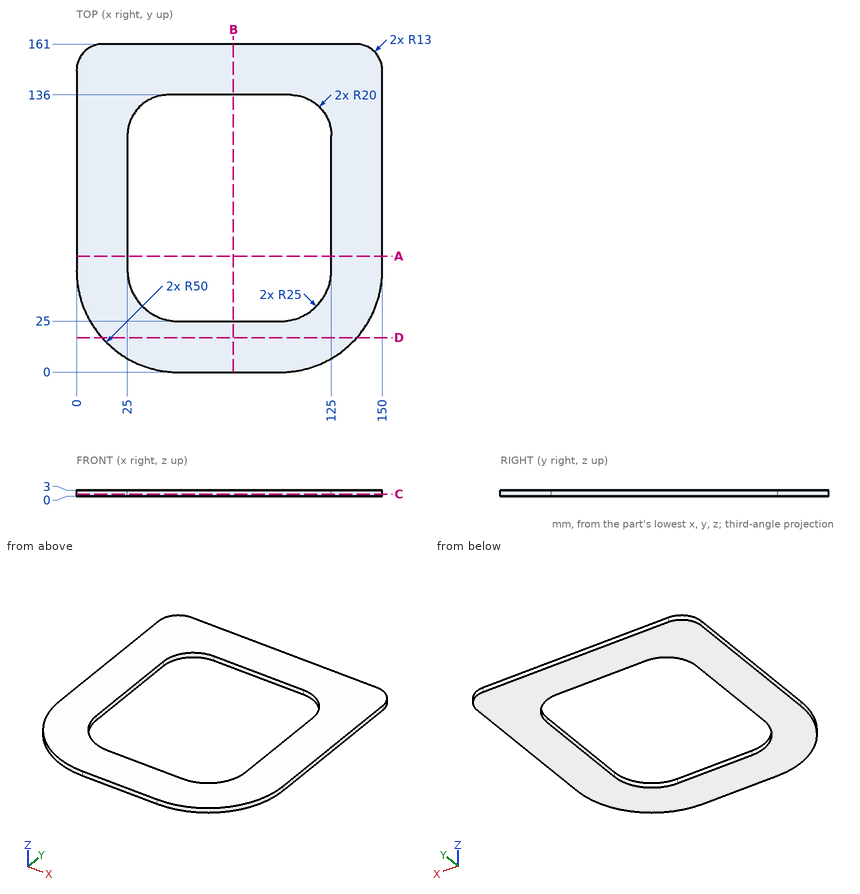
Here's the drawing with two shaded views (mm, measured from the low corner). I have some questions. Coordinates: 2 decimals unless noted, no trailing zeros. Write each loop counter-clockwise with the first axis right and the second up, starting at its lowest first coordinate (ties: lowest second). Pieces come first, ordered by that corner, then holes.
Item 1: I want a section at A-A on y = 57. Write out the boundary of the cut face in (x, z), and give its area (3 significant figures).
Item 2: I want a section at D-D on y = 17. Write out the boundary of the cut face in (x, z).
Item 3: I want a section at B-B on x = 77. Write out the boundary of the cut face in (y, z), and give its area (3 significant figures).
Item 4: If I drill on line 1 (Y direction, x = 62, z = 0.3); line 2 (X direction, y = 62.5, z = 0.3); line 3 (X direction, y = 31, z = 2.3), over which ranges is the centre line in solid material (lowest first)?
Item 5: I want a section at C-C on z = 1.05. Write out the boundary of the cut face in (x, y).
Findings below:
1. outline: (0, 0) - (25, 0) - (25, 3) - (0, 3) - close; (125, 0) - (150, 0) - (150, 3) - (125, 3) - close
1. area: 150 mm2
2. outline: (12.44, 0) - (137.56, 0) - (137.56, 3) - (12.44, 3) - close
3. outline: (0, 0) - (25, 0) - (25, 3) - (0, 3) - close; (136, 0) - (161, 0) - (161, 3) - (136, 3) - close
3. area: 150 mm2
4. line 1: y = 0 to 25, 136 to 161
4. line 2: x = 0 to 25, 125 to 150
4. line 3: x = 3.75 to 33.75, 116.25 to 146.25
5. outline: (0, 50) arc R50 ccw to (50, 0) - (100, 0) arc R50 ccw to (150, 50) - (150, 148) arc R13 ccw to (137, 161) - (13, 161) arc R13 ccw to (0, 148) - close; hole (25, 50) arc R25 ccw to (50, 25) - (100, 25) arc R25 ccw to (125, 50) - (125, 116) arc R20 ccw to (105, 136) - (45, 136) arc R20 ccw to (25, 116) - close
